Build history of the part. All positions in model axes, mm. A direction names the side the tool comes from. Coordinates: 2 decimals unless noted, no trailing zeros. Order: outer loops, then holes, each group sorted by start corner. A loop starts at its lowest first (then second) coordinate and runs counter-clockwise, first axis right, second up. Notation, with made-up numbers: (-20.5, -18) -> (14.5, -18) arc R17 cw to (14.5, -5) -> close; hole circle Ø5 at (-36.75, 33). An arc over 180 degrees is marked (long way). Write each question's results on one line, items separated by ' | '.
from build123d import *

# Parameters (mm, degrees)
CROQUIS8_W                   = 6
CROQUIS8_H                   = 126
CROQUIS8_W_2                 = 60
CROQUIS8_H_2                 = 8
SALIENTE_EXTRUIR1_DEPTH      = 8
TALADRO_DE_MARGEN_PARA_M31_D = 3.6
TALADRO_DE_MARGEN_PARA_M32_D = 3.6


with BuildPart() as part:
    # Croquis8 → Saliente-Extruir1 (new body)
    with BuildSketch(Plane.XY):
        Polygon((7.730954987, 134), (13.730954987, 134), (13.730954987, 142), (-2.269045013, 142), (-2.269045013, 134), align=None)
        with Locations((10.730954987, 71)):
            Rectangle(CROQUIS8_W, CROQUIS8_H)
        Polygon((41.730954987, 142), (41.730954987, 134), (47.730954987, 134), (57.730954987, 134), (57.730954987, 142), align=None)
        with Locations((44.730954987, 71)):
            Rectangle(CROQUIS8_W, CROQUIS8_H)
        with Locations((30, 4)):
            Rectangle(CROQUIS8_W_2, CROQUIS8_H_2)
    extrude(amount=SALIENTE_EXTRUIR1_DEPTH)

    # Taladro de margen para M31 (through all)
    with Locations(Plane(origin=(57.730954987, 0, 0), x_dir=(0, 0, -1), z_dir=(1, 0, 0))):
        with Locations((-4, 138)):
            Hole(TALADRO_DE_MARGEN_PARA_M31_D / 2)

    # Taladro de margen para M32 (through all)
    with Locations(Plane(origin=(60, 0, 0), x_dir=(0, 0, -1), z_dir=(1, 0, 0))):
        with Locations((-4, 4)):
            Hole(TALADRO_DE_MARGEN_PARA_M32_D / 2)


solid = part.part
Item 1: Slice it at D-D, the plane z = 4. List the corners of the cut face in (x, y).
Answer:
outline: (-2.27, 134) -> (7.73, 134) -> (7.73, 8) -> (0, 8) -> (0, 5.8) -> (60, 5.8) -> (60, 8) -> (47.73, 8) -> (47.73, 134) -> (57.73, 134) -> (57.73, 136.2) -> (41.73, 136.2) -> (41.73, 8) -> (13.73, 8) -> (13.73, 136.2) -> (-2.27, 136.2) -> close; (-2.27, 139.8) -> (13.73, 139.8) -> (13.73, 142) -> (-2.27, 142) -> close; (0, 0) -> (60, 0) -> (60, 2.2) -> (0, 2.2) -> close; (41.73, 139.8) -> (57.73, 139.8) -> (57.73, 142) -> (41.73, 142) -> close
Item 2: Tool access for faces 5 (the flat face through (54, 8, 4)), 6 (the flat face through (7.731, 70, 4)), 7 (the flat face through (57.731, 138, 2)), 8 (the flat face through (41.731, 76, 4)): list every direction of +Z, -Z, +X, -X, +Y, -Y with a clear straight run to the whole face (end or side of a thin tool).
Answer:
face 5: +Z, -Z, +X | face 6: +Z, -Z, -X | face 7: +Z, -Z, +X, +Y | face 8: +Z, -Z, +Y
Item 3: Slice it at B-B, the plane x = 49. List the corners of the cut face in (y, z).
Answer:
outline: (0, 0) -> (8, 0) -> (8, 8) -> (0, 8) -> close; (134, 0) -> (142, 0) -> (142, 8) -> (134, 8) -> close; hole circle Ø3.6 at (4, 4); hole circle Ø3.6 at (138, 4)
Item 4: Slice it at C-C, the plane y = 138. List the corners of the cut face in (x, z).
Answer:
outline: (-2.27, 0) -> (13.73, 0) -> (13.73, 2.2) -> (-2.27, 2.2) -> close; (-2.27, 5.8) -> (13.73, 5.8) -> (13.73, 8) -> (-2.27, 8) -> close; (41.73, 0) -> (57.73, 0) -> (57.73, 2.2) -> (41.73, 2.2) -> close; (41.73, 5.8) -> (57.73, 5.8) -> (57.73, 8) -> (41.73, 8) -> close
Item 5: Pin check, flat tips, straight feed: pin 1 (2.5 mm diameter, centred on y = 138.5, z = 2, fed in from +X); pin 2 (2 mm diameter, centred on x = 17.5, z = 4.5, fed in from -Y); pin 3 (2.5 mm diameter, centred on x = 29, z = 4, fed in from +Y); pin 4 (2 mm diameter, centred on y = 87.5, z = 3, fed in from +X). Stop position of each tip, or through.
Answer:
pin 1: stops at x = 57.73 | pin 2: stops at y = 0 | pin 3: stops at y = 8 | pin 4: stops at x = 47.73
Item 6: Slice it at A-A, the plane y = 79. List the corners of the cut face in (x, z), and give its area (3 significant figures).
Answer:
outline: (7.73, 0) -> (13.73, 0) -> (13.73, 8) -> (7.73, 8) -> close; (41.73, 0) -> (47.73, 0) -> (47.73, 8) -> (41.73, 8) -> close | area: 96.0 mm^2
Item 7: Pull direction Y, two halves, no side cores. Call faces 1 (the flat face through (53, 134, 4)), 2 (the flat face through (0, 4, 2)), 3 (the flat face through (47.731, 70, 4)), 4 (the flat face through (6, 142, 4)): released by +Y, released by -Y, zero draft, split by the parting line, or undercut.
Answer:
face 1: undercut | face 2: zero draft | face 3: undercut | face 4: released by +Y
Item 8: Drill centre lines: line 1 (Y direction, x = 13, z = 4); line 2 (Y direction, x = 51, z = 4); line 3 (X direction, y = 107, z = 3). Where is each one in solid material? Low to high. Write a range as from..to.
Answer:
line 1: y = 0..2.2, 5.8..136.2, 139.8..142 | line 2: y = 0..2.2, 5.8..8, 134..136.2, 139.8..142 | line 3: x = 7.73..13.73, 41.73..47.73
